```python
from build123d import *

# Parameters (mm, degrees)
SKETCH1_W                      = 192.96
SKETCH1_H                      = 110.76
BOSS_EXTRUDE1_DEPTH            = 5
CBORE_START                    = 2
CBORE_FOR_M3_SHCS1_OUTLINE_R   = 3.25
CBORE_FOR_M3_SHCS1_DEPTH       = 3
CBORE_FOR_M3_SHCS1_2_OUTLINE_R = 1.8
CBORE_FOR_M3_SHCS1_2_DEPTH     = 2
SKETCH9_W                      = 21
SKETCH9_H                      = 16
CUT_EXTRUDE1_DEPTH             = 112.356790543
FILLET1_R                      = 10
FILLET2_R                      = 10
FILLET3_R                      = 1


# Read off the part's stored shape, not the designer's step: CBORE for M3 SHCS1
with BuildPart() as part:
    # Sketch1 → Boss-Extrude1 (new body)
    with BuildSketch(Plane(origin=(0, 0, 0), x_dir=(1, 0, 0), z_dir=(0, 1, 0))):
        Rectangle(SKETCH1_W, SKETCH1_H)
    extrude(amount=BOSS_EXTRUDE1_DEPTH)

    # CBORE for M3 SHCS1 outline → CBORE for M3 SHCS1 (cut)
    with BuildSketch(Plane(origin=(0, 0, 0), x_dir=(1, 0, 0), z_dir=(0, 1, 0)).offset(CBORE_START)):
        with Locations((63.1, -32.825)):
            Circle(CBORE_FOR_M3_SHCS1_OUTLINE_R)
        with Locations((-63.1, 32.825)):
            Circle(CBORE_FOR_M3_SHCS1_OUTLINE_R)
        with Locations((-63.1, -32.825)):
            Circle(CBORE_FOR_M3_SHCS1_OUTLINE_R)
        with Locations((63.1, 32.825)):
            Circle(CBORE_FOR_M3_SHCS1_OUTLINE_R)
    extrude(amount=CBORE_FOR_M3_SHCS1_DEPTH, mode=Mode.SUBTRACT)

    # CBORE for M3 SHCS1 2 outline → CBORE for M3 SHCS1 2 (cut)
    with BuildSketch(Plane(origin=(0, 0, 0), x_dir=(1, 0, 0), z_dir=(0, 1, 0))):
        with Locations((63.1, -32.825)):
            Circle(CBORE_FOR_M3_SHCS1_2_OUTLINE_R)
        with Locations((-63.1, 32.825)):
            Circle(CBORE_FOR_M3_SHCS1_2_OUTLINE_R)
        with Locations((-63.1, -32.825)):
            Circle(CBORE_FOR_M3_SHCS1_2_OUTLINE_R)
        with Locations((63.1, 32.825)):
            Circle(CBORE_FOR_M3_SHCS1_2_OUTLINE_R)
    extrude(amount=CBORE_FOR_M3_SHCS1_2_DEPTH, mode=Mode.SUBTRACT)

    # Sketch9 → Cut-Extrude1 (cut, through all)
    with BuildSketch(Plane(origin=(0, 5, 0), x_dir=(1, 0, 0), z_dir=(0, 1, 0))):
        Polygon((45.98, 10.38), (28.98, 10.38), (28.98, -11.62), (14.6, -11.62), (14.6, -42.38), (37.6, -42.38), (37.6, -15.62), (45.98, -15.62), (45.98, -12.62), (63.1, -12.62), (63.1, 7.38), (45.98, 7.38), align=None)
        with Locations((-20, 11)):
            Rectangle(SKETCH9_W, SKETCH9_H)
    extrude(amount=-CUT_EXTRUDE1_DEPTH, mode=Mode.SUBTRACT)

    # Fillet1
    fillet1_edges = [part.edges().sort_by_distance(p)[0] for p in [
        (-96.48, 2.5, -55.38),
        (96.48, 2.5, -55.38),
        (96.48, 2.5, 55.38),
        (-96.48, 2.5, 55.38),
    ]]
    fillet(fillet1_edges, radius=FILLET1_R)

    # Fillet2
    # the kernel refuses this fillet: 10 mm, written as the material it takes off along each edge
    with BuildSketch(Plane(origin=(37.6, 29.669768949, 15.62), x_dir=(1, 0, 0), z_dir=(0, -1, 0))) as fillet2_piece_1:
        with BuildLine():
            CenterArc((10, 9.86790758), FILLET2_R, 180, 80.676997523)
            Line((0, 9.86790758), (-0.2, 9.86790758))
            Line((-0.2, 9.86790758), (-0.2, 0))
            Line((-0.2, 0), (0, -0.2))
            ThreePointArc((0, -0.2), (4.19, -0.2), (8.3476, -0.197358152))
            Line((8.3476, -0.197358152), (8.38, 0))
        make_face()
    extrude(amount=54.339537898, mode=Mode.SUBTRACT)
    with BuildSketch(Plane(origin=(28.98, 30, 11.62), x_dir=(-1, 0, 0), z_dir=(0, -1, 0))) as fillet2_piece_2:
        with BuildLine():
            CenterArc((FILLET2_R, FILLET2_R), FILLET2_R, 180, 90)
            Line((0, FILLET2_R), (-FILLET2_R * 0.02, FILLET2_R))
            Line((-FILLET2_R * 0.02, FILLET2_R), (-FILLET2_R * 0.02, -FILLET2_R * 0.02))
            Line((-FILLET2_R * 0.02, -FILLET2_R * 0.02), (FILLET2_R, -FILLET2_R * 0.02))
            Line((FILLET2_R, -FILLET2_R * 0.02), (FILLET2_R, 0))
        make_face()
    extrude(amount=55, mode=Mode.SUBTRACT)

    # Fillet3
    fillet3_edges = [part.edges().sort_by_distance(p)[0] for p in [
        (-30.5, 2.5, -3),
        (-30.5, 2.5, -19),
        (-9.5, 2.5, -19),
        (-9.5, 2.5, -3),
        (45.98, 2.5, -10.38),
        (45.98, 2.5, -7.38),
        (63.1, 2.5, -7.38),
        (63.1, 2.5, 12.62),
        (45.98, 2.5, 12.62),
        (45.98, 2.5, 15.62),
        (37.6, 2.5, 42.38),
        (14.6, 2.5, 42.38),
        (14.6, 2.5, 11.62),
        (28.98, 2.5, -10.38),
    ]]
    fillet(fillet3_edges, radius=FILLET3_R)


solid = part.part
```
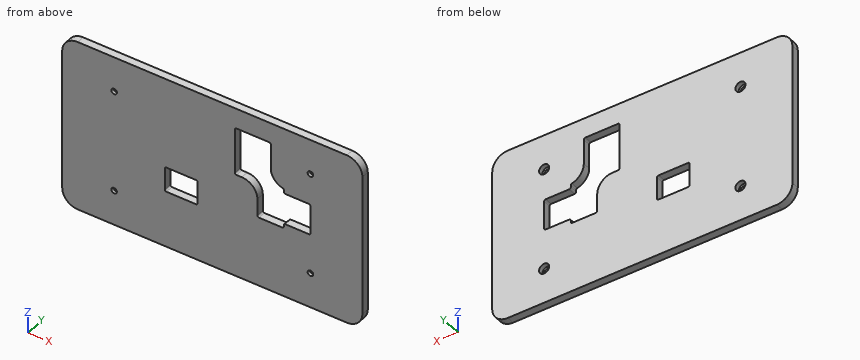
Model file for the job. Use its own axes, mm. Give positions to 0.01 mm unless a question says otherwise; leave off trailing zeros. Order: outer loops, then holes, each group sorted by start corner. A loop starts at its lowest first (then second) coordinate and runs counter-clockwise, first axis right, second up.
1) Saw through at D-D, the plane y = 2.9. Count the separate pieces of the cut face and the enclosed holes in it, then the cut area to 3 significant figures.
2) Saw through at B-B, the plane z = 27.5. Write the cut outline in (x, y), then the cut area to 3 significant figures.
3) Wall check: probe 1 along Z at (x, y) = (-63.1, 0.5) (3 decimals); probe 2 along X at (y, z) = (3.95, 37.5); probe 3 along Z at (x, y) = (-21.5, 3.4). Give the ranges that are in metal, low to high.
4) Saw through at C-C, the plane x = -18.5. Write the cut outline in (y, z).
5) Pin check, flat tip, straight feed: pin 1 (4.5 mm diameter, centred on x = -63.1, z = -32.825, fed in from +Y). Stop position of the tip, or through.
6) Saw through at A-A, the plane x = -63.1. Write the cut outline in (y, z) (3 decimals).
Computed:
1. separate pieces: 1
1. enclosed holes: 6
1. area: 19,300 mm2
2. outline: (-96.48, 0) - (14.6, 0) - (14.6, 5) - (-96.48, 5) - close; (37.6, 0) - (96.48, 0) - (96.48, 5) - (37.6, 5) - close
2. area: 850 mm2
3. probe 1: z = -55.38 to -34.625, -31.025 to 31.025, 34.625 to 55.38
3. probe 2: x = -96.48 to 14.6, 37.6 to 96.48
3. probe 3: z = -55.38 to -19, -3 to 55.38
4. outline: (0, -55.38) - (5, -55.38) - (5, -19) - (0, -19) - close; (0, -3) - (5, -3) - (5, 55.38) - (0, 55.38) - close
5. pin 1: stops at y = 2
6. outline: (0, -55.38) - (5, -55.38) - (5, -36.075) - (2, -36.075) - (2, -34.625) - (0, -34.625) - close; (0, -31.025) - (2, -31.025) - (2, -29.575) - (5, -29.575) - (5, 29.575) - (2, 29.575) - (2, 31.025) - (0, 31.025) - close; (0, 34.625) - (2, 34.625) - (2, 36.075) - (5, 36.075) - (5, 55.38) - (0, 55.38) - close
